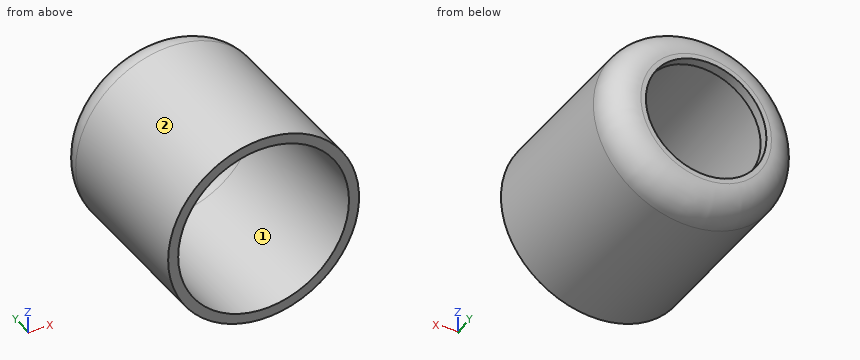
Autodesk Inventor part; units mm, degrees
ref_plane "YZ Plane" through (0, 0, 0) normal (1, 0, 0) x (0, 1, 0)
ref_plane "XZ Plane" through (0, 0, 0) normal (0, 1, 0) x (-1, 0, 0)
ref_plane "XY Plane" through (0, 0, 0) normal (0, 0, 1) x (1, 0, 0)
sketch "Sketch1" plane through (0, 0, 0) normal (0, 0, 1) x (1, 0, 0)
  line L0 (11.5, 9) -> (11.5, 6) construction
  arc A0 (11.5, 6) -> (13.5, 6) centre (12.5, 6) ccw construction
  line L1 (13.5, 6) -> (13.5, 19.8063) construction
  arc A1 (13.5, 19.8063) -> (12, 21.3063) centre (12, 19.8063) ccw construction
  arc A2 (12, 24.3063) -> (12, 21.3063) centre (12, 22.8063) ccw construction
  arc A3 (12, 24.3063) -> (13.5, 25.8063) centre (12, 25.8063) ccw construction
  line L2 (13.5, 25.8063) -> (13.5, 71) construction
  arc A4 (13.5, 71) -> (11.5, 73) centre (11.5, 71) ccw construction
  line L3 (11.5, 73) -> (2, 73) construction
  line L4 (2, 73) -> (2, 80) construction
  arc A5 (2, 80) -> (1.2, 81.6) centre (0, 80) ccw construction
  arc A6 (0, 84) -> (1.2, 81.6) centre (3, 84) ccw construction
  arc A7 (-1.2, 81.6) -> (0, 84) centre (-3, 84) ccw construction
  arc A8 (-1.2, 81.6) -> (-2, 80) centre (0, 80) ccw construction
  line L5 (-2, 80) -> (-2, 73) construction
  line L6 (-2, 73) -> (-11.5, 73) construction
  arc A9 (-11.5, 73) -> (-13.5, 71) centre (-11.5, 71) ccw construction
  line L7 (-13.5, 71) -> (-13.5, 25.8063) construction
  arc A10 (-13.5, 25.8063) -> (-12, 24.3063) centre (-12, 25.8063) ccw construction
  arc A11 (-12, 21.3063) -> (-12, 24.3063) centre (-12, 22.8063) ccw construction
  arc A12 (-12, 21.3063) -> (-13.5, 19.8063) centre (-12, 19.8063) ccw construction
  line L8 (-13.5, 19.8063) -> (-13.5, 6) construction
  arc A13 (-13.5, 6) -> (-11.5, 6) centre (-12.5, 6) ccw construction
  line L9 (-11.5, 6) -> (-11.5, 9) construction
  arc A14 (-9.5, 11) -> (-11.5, 9) centre (-9.5, 9) ccw construction
  line L10 (-9.5, 11) -> (-9.5, 6) construction
  arc A15 (-15.5, 6) -> (-9.5, 6) centre (-12.5, 6) ccw construction
  line L11 (-15.5, 6) -> (-15.5, 19.8063) construction
  arc A16 (-13.8028, 22.8063) -> (-15.5, 19.8063) centre (-12, 19.8063) ccw construction
  arc A17 (-15.5, 25.8063) -> (-13.8028, 22.8063) centre (-12, 25.8063) ccw construction
  line L12 (-15.5, 25.8063) -> (-15.5, 71) construction
  arc A18 (-11.5, 75) -> (-15.5, 71) centre (-11.5, 71) ccw construction
  line L13 (-11.5, 75) -> (-3, 75) construction
  line L14 (-3, 75) -> (-3, 80) construction
  arc A19 (-1.8, 82.4) -> (-3, 80) centre (0, 80) ccw construction
  arc A20 (-1.8, 82.4) -> (-1, 84) centre (-3, 84) ccw construction
  arc A21 (0, 85) -> (-1, 84) centre (0, 84) ccw construction
  arc A22 (1, 84) -> (0, 85) centre (0, 84) ccw construction
  arc A23 (1, 84) -> (1.8, 82.4) centre (3, 84) ccw construction
  arc A24 (3, 80) -> (1.8, 82.4) centre (0, 80) ccw construction
  line L15 (3, 80) -> (3, 75) construction
  line L16 (3, 75) -> (11.5, 75) construction
  arc A25 (15.5, 71) -> (11.5, 75) centre (11.5, 71) ccw construction
  line L17 (15.5, 71) -> (15.5, 25.8063) construction
  arc A26 (13.8028, 22.8063) -> (15.5, 25.8063) centre (12, 25.8063) ccw construction
  arc A27 (15.5, 19.8063) -> (13.8028, 22.8063) centre (12, 19.8063) ccw construction
  line L18 (15.5, 19.8063) -> (15.5, 6) construction
  arc A28 (9.5, 6) -> (15.5, 6) centre (12.5, 6) ccw construction
  line L19 (9.5, 6) -> (9.5, 11) construction
  arc A29 (11.5, 9) -> (9.5, 11) centre (9.5, 9) ccw construction
  line L20 (-9.5, 6) -> (-8.5, 6)
  line L21 (-8.5, 6) -> (-8.5, 22)
  line L22 (-9.5, 22) -> (-9.5, 6)
  arc A30 (-6.5, 25) -> (-9.5, 22) centre (-6.5, 22) ccw
  arc A31 (-6.5, 24) -> (-8.5, 22) centre (-6.5, 22) ccw
  line L23 (-6, 25) -> (-6.5, 25)
  line L24 (-6, 24) -> (-6.5, 24)
  line L25 (5.1354, 22) -> (-7.1821, 22) construction
  line L26 (0, 22) -> (0, 0) construction
  line L27 (-6, 25) -> (-6, 24)
  dimension "d0" = 1
  dimension "d2" = 18
  dimension "d3" = 6
  dimension "d4" = 2
  dimension "d5" = 6
revolve "Revolution1" add sketch "Sketch1" angle 360 about axis through (0, 22, 0) along (0, -1, 0)
equation "\"d0\" = d1"
properties part number "anode-bell" material "Stainless Steel"
Input: part model. Units: mm. Frame: model coordinates. Face numbers are marked on the shaded views. A direction names the side the tool comes from. Round coordinates to 2 decimals unless told otherwise and drop trailing zeros. Loops run counter-clockwise (first coordinate to the right, second up) from the corner with the lowest first, then second, coordinate; pieces in that order, holes last. Notation, with made-up numbers: (-35.75, 47) -> (14.25, 47) arc R27 cw to (14.25, 63) -> close; hole circle Ø1 at (-34, 29.5). An arc over 180 degrees is marked (long way). Answer as a JSON object with one key per item and string values. Group by question number.
1) Reachability of the marked faces 1 and 2 from +Z, -Z, +X, -X, +Y, -Y: full face, straight path, thin tool, end or side. Return the list, or none.
2) Ray query, L1, parallel to Z at x = 0, y = 18; L2, parallel to X at y = 24.25, z = 0. Return the intervals inside material, ascending.
3) Section query B-B on x = 0. Output: boundary loops of the cut face in (y, z), plus the area to 3 significant figures.
4) Section query C-C on y = 20.5. Output: boundary loops of the cut face in (x, z).
5) Section query A-A on z = 0. Output: boundary loops of the cut face in (x, y).
6) Pin query (flat end, axial travel): pin 1 (3 mm diameter, centred on x = 4.5, y = 12.5, fed in from -Z); pin 2 (5 mm diameter, centred on y = 21.5, z = 2.5, fed in from +X); pin 3 (5 mm diameter, centred on y = 10.5, z = 6, fed in from -X); pin 4 (1 mm diameter, centred on x = 5.5, y = 22, fed in from -Z). Return the tip coordinate at first contact, or that it passes through.
Reply:
{
 "1": {"face 1": "-Y", "face 2": "+Y, -Y"},
 "2": {"L1": "z = -9.5 to -8.5, 8.5 to 9.5", "L2": "x = -8.48 to -6, 6 to 8.48"},
 "3": {"outline": "(6, -9.5) -> (22, -9.5) arc R3 ccw to (25, -6.5) -> (25, -6) -> (24, -6) -> (24, -6.5) arc R2 cw to (22, -8.5) -> (6, -8.5) -> close; (6, 8.5) -> (22, 8.5) arc R2 cw to (24, 6.5) -> (24, 6) -> (25, 6) -> (25, 6.5) arc R3 ccw to (22, 9.5) -> (6, 9.5) -> close", "area": "40.9 mm2"},
 "4": {"outline": "circle Ø19 at (0, 0); hole circle Ø17 at (0, 0)"},
 "5": {"outline": "(-9.5, 6) -> (-8.5, 6) -> (-8.5, 22) arc R2 cw to (-6.5, 24) -> (-6, 24) -> (-6, 25) -> (-6.5, 25) arc R3 ccw to (-9.5, 22) -> close; (6, 24) -> (6.5, 24) arc R2 cw to (8.5, 22) -> (8.5, 6) -> (9.5, 6) -> (9.5, 22) arc R3 ccw to (6.5, 25) -> (6, 25) -> close"},
 "6": {"pin 1": "stops at z = -9.01", "pin 2": "stops at x = 9.5", "pin 3": "stops at x = -8.83", "pin 4": "stops at z = -8.08"}
}
